Study the drawing (mm; zero at the part's minimum x, y, z) and answer. Round coordinates to 2 decimals unless told otherwise and drop trailing zeros. Loops run counter-clockwise (first coordinate to the right, second up) from the corner with the lowest first, then second, coordinate; pieces in that order, holes last. Notation, with made-up numbers: (87, -11.75) - (103, -11.75) arc R12 ccw to (103, -7.75) - close; hole circle Ø6 at (-13, 31). An arc over 180 degrees is marked (long way). One line per item, written item: value.
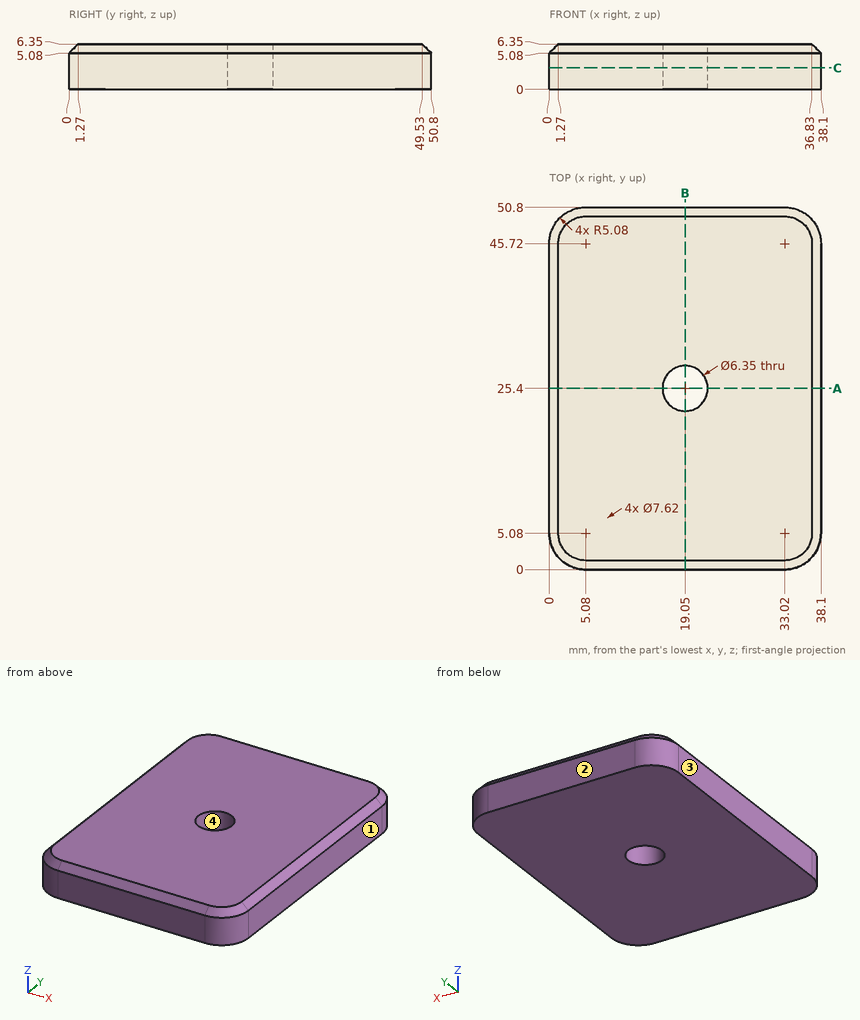
1) A cutting plane is placed at B-B on x = 19.05. Give the vertices of the cut face in (y, z) (3 decimals).
Final values:
outline: (0, 0) - (22.225, 0) - (22.225, 6.35) - (1.27, 6.35) - (0, 5.08) - close; (28.575, 0) - (50.8, 0) - (50.8, 5.08) - (49.53, 6.35) - (28.575, 6.35) - close
2) For a pull along X with two mould halves and no side action, classify the marked faces 1, 2, 3 and 4 as released by +X, released by -X, zero draft, split by the parting line, or undercut.
Final values:
face 1: released by +X
face 2: zero draft
face 3: released by -X
face 4: undercut
3) A cutting plane is placed at C-C on z = 3. Give the vertices of the cut face in (x, y) (3 decimals), and give its area (3 significant figures).
Final values:
outline: (0, 5.08) arc R5.08 ccw to (5.08, 0) - (33.02, 0) arc R5.08 ccw to (38.1, 5.08) - (38.1, 45.72) arc R5.08 ccw to (33.02, 50.8) - (5.08, 50.8) arc R5.08 ccw to (0, 45.72) - close; hole circle Ø6.35 at (19.05, 25.4)
area: 1,880 mm2
4) Consider L1, parallel to Y at x = 19.05, z = 3.5 (3 decimals); L2, parallel to Y at x = 5, z = 4.25; L3, parallel to Y at x = 20.5, z = 2. Determine where each line is inside the solid, lowest interval first.
Final values:
L1: 0 to 22.225, 28.575 to 50.8
L2: 0 to 50.8
L3: 0 to 22.58, 28.22 to 50.8
5) A cutting plane is placed at A-A on y = 25.4. Give the vertices of the cut face in (x, z) (3 decimals).
Final values:
outline: (0, 0) - (15.875, 0) - (15.875, 6.35) - (1.27, 6.35) - (0, 5.08) - close; (22.225, 0) - (38.1, 0) - (38.1, 5.08) - (36.83, 6.35) - (22.225, 6.35) - close
